```python
from build123d import *

# Parameters (mm, degrees)
SKETCH077_W     = 33
SKETCH077_H     = 12
SKETCH077_R     = 1.75
PAD042_DEPTH    = 5
POCKET029_DEPTH = 3
SKETCH079_R     = 3.6
POCKET030_DEPTH = 5


with BuildPart() as part:
    # Sketch077 → Pad042 (new body)
    with BuildSketch(Plane.YZ):
        with Locations((16.5, 6)):
            Rectangle(SKETCH077_W, SKETCH077_H)
        with Locations((2.5, 9.5)):
            Circle(SKETCH077_R, mode=Mode.SUBTRACT)
        with Locations((2.5, 2.5)):
            Circle(SKETCH077_R, mode=Mode.SUBTRACT)
        with Locations((30.5, 9.5)):
            Circle(SKETCH077_R, mode=Mode.SUBTRACT)
        with Locations((30.5, 2.5)):
            Circle(SKETCH077_R, mode=Mode.SUBTRACT)
    extrude(amount=PAD042_DEPTH)

    # Sketch078 → Pocket029 (cut)
    with BuildSketch(Plane(origin=(0, 9, 6), x_dir=(0, 0, -1), z_dir=(1, 0, 0))):
        with BuildLine():
            ThreePointArc((-3.584145, 0.3375), (0, -3.6), (3.584145, 0.3375))
            Line((2.090751, 16.196875), (3.584145, 0.3375))
            ThreePointArc((2.090751, 16.196875), (0, 18.1), (-2.090751, 16.196875))
            Line((-2.090751, 16.196875), (-3.584145, 0.3375))
        make_face()
    extrude(amount=POCKET029_DEPTH, mode=Mode.SUBTRACT)

    # Sketch079 → Pocket030 (cut)
    with BuildSketch(Plane(origin=(0, 9, 6), x_dir=(0, 1, 0), z_dir=(1, 0, 0))):
        Circle(SKETCH079_R)
    extrude(amount=POCKET030_DEPTH, mode=Mode.SUBTRACT)


with BuildPart() as part_1:
    # Body012 placement: moved
    add(part.part.moved(Location((10, -22, 16.4))))


solid = part_1.part
```
CAD build for the part. Positions are in the model's coordinates, mm. A direction names the side the tool comes from. Round coordinates to 2 decimals unless told otherwise and drop trailing zeros. Write each loop counter-clockwise with the first axis right and the second up, starting at its lowest first coordinate (ties: lowest second). Pieces come first, ordered by that corner, then holes. Notation, with made-up numbers: (-10, 28) - (-3, 28) arc R24 cw to (-3, 52) - close; hole circle Ø8 at (85, 7.5). An arc over 180 degrees is marked (long way). Return JSON: item names as keys, results as strings. Group by question number.
Item 1: Probe probe 1 along Z at (x, y) = (13.35, 8.5); probe 2 along Y at (x, z) = (13.1, 18.5); probe 3 along Y at (x, z) = (13.6, 17.75). List the from-to ranges inside material, lowest first.
Item 2: Band-saw the part on D-D on z = 22.4. List the corners of the cut face in (x, y).
Item 3: Band-saw the part on A-A on y = -13. List the corners of the cut face in (x, z).
Item 4: Band-saw the part on B-B on x = 11.4. List the corners of the cut face in (y, z).
Item 5: Flat gauge pins, fed straight in: pin 1 Ø4.5 at (y, z) = (-19.5, 18.9) entering from +X; pin 2 Ø6 at (y, z) = (-13, 22.4) entering from +X; pin 3 Ø2 at (y, z) = (-6.5, 23) entering from -X. Where does each tip first touch, or does it go through?
Item 6: Mould opens along Y. For faces 3 (the face through (12, -6, 16.4)), 4 (the face through (12, -21, 18)), 5 (the face through (12, -22, 22)), 6 (the face through (12, 11, 22)) say: +Y half, -Y half, draft (parallel to the pull), parting line (faces both ways), or undercut.
Item 7: Band-saw the part on C-C on y = 8.5. List the corners of the cut face in (x, z), plus the area to 3 significant figures.
Item 8: 3-axis set-ups, long thin cutter, end or side, ignore diameter. For faces 1 (the face through (13, -4, 22)), 2 (the face through (12.46, 8.12, 24.19)): which of +Z, -Z, +X, -X, +Y, -Y reach the whole face in a straight line?
Resolved:
{
 "1": {"probe 1": "z = 16.4 to 17.15, 20.65 to 24.15, 27.65 to 28.4", "probe 2": "y = -22 to -21.2, -17.8 to 6.8, 10.2 to 11", "probe 3": "y = -22 to -20.82, -18.18 to 7.18, 9.82 to 11"},
 "2": {"outline": "(10, -22) - (15, -22) - (15, -16.6) - (10, -16.6) - close; (10, 5.1) - (13, 5.1) - (13, -9.4) - (15, -9.4) - (15, 11) - (10, 11) - close"},
 "3": {"outline": "(10, 16.4) - (15, 16.4) - (15, 18.8) - (10, 18.8) - close; (10, 26) - (15, 26) - (15, 28.4) - (10, 28.4) - close"},
 "4": {"outline": "(-22, 16.4) - (11, 16.4) - (11, 28.4) - (-22, 28.4) - close; hole circle Ø3.5 at (-19.5, 18.9); hole circle Ø3.5 at (-19.5, 25.9); hole (-12.66, 18.82) - (3.2, 20.31) arc R2.1 ccw to (3.2, 24.49) - (-12.66, 25.98) arc R3.6 ccw (long way) to start; hole circle Ø3.5 at (8.5, 18.9); hole circle Ø3.5 at (8.5, 25.9)"},
 "5": {"pin 1": "stops at x = 15", "pin 2": "passes through", "pin 3": "stops at x = 13"},
 "6": {"face 3": "draft", "face 4": "undercut", "face 5": "-Y half", "face 6": "+Y half"},
 "7": {"outline": "(10, 16.4) - (15, 16.4) - (15, 17.15) - (10, 17.15) - close; (10, 20.65) - (15, 20.65) - (15, 24.15) - (10, 24.15) - close; (10, 27.65) - (15, 27.65) - (15, 28.4) - (10, 28.4) - close", "area": "25.0 mm²"},
 "8": {"face 1": "-X", "face 2": "+X, -X"}
}
